Print and shaded views of the part. All mm, measured from the part's lowest x, y and z. Round coordinates to 2 decimals unless told otherwise and drop trailing zeros. Loops run counter-clockwise (first coordinate to the right, second up) from the corner with the lowest first, then second, coordinate; pieces in that order, holes last. Notation, with made-up numbers: (46, 6.5) - (93, 6.5) arc R25 cw to (93, 41.5) - close; hole circle Ø1 at (42, 2). An arc over 180 degrees is marked (long way). Use one line per item in the form item = value. Start each with the question number.
Q1. Saw through at B-B (y = 9.5). Give the cut face in (x, z), then the cut area to 3 significant figures.
Q2. Saw through at A-A (z = 37). Give the cut face in (x, y).
Q3. Saw through at C-C (x = 10). Give the cut face in (y, z), then the cut area to 3 significant figures.
Q4. Drill centre lines: line 1 (Z direction, x = 10, y = 5); line 2 (Z direction, x = 8.5, y = 9.25); line 3 (Z direction, x = 18.25, y = 8.75). Where is each one in solid material? Low to high.
Q5. Pin check, flat tips, straight feed: pin 1 (5 mm diameter, centred on y = 3, z = 33.5, fed in from -X); pin 2 (3.5 mm diameter, centred on x = 10, z = 37, fed in from +Y). Stop position of each tip, or through.
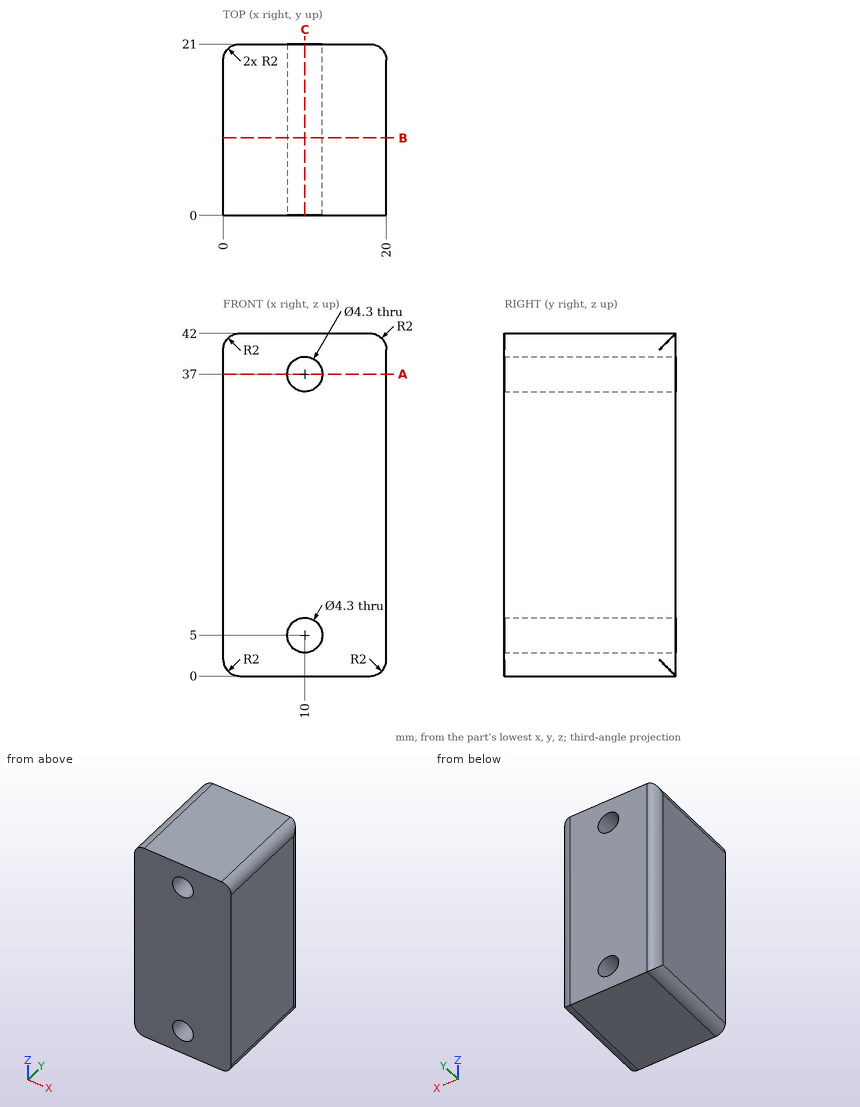
Report:
q1.outline = (0, 2) arc R2 ccw to (2, 0) - (18, 0) arc R2 ccw to (20, 2) - (20, 40) arc R2 ccw to (18, 42) - (2, 42) arc R2 ccw to (0, 40) - close; hole circle Ø4.3 at (10, 5); hole circle Ø4.3 at (10, 37)
q1.area = 808 mm²
q2.outline = (0, 0) - (7.85, 0) - (7.85, 21) - (2, 21) arc R2 ccw to (0, 19) - close; (12.15, 0) - (20, 0) - (20, 19) arc R2 ccw to (18, 21) - (12.15, 21) - close
q3.outline = (0, 0) - (21, 0) - (21, 2.85) - (0, 2.85) - close; (0, 7.15) - (21, 7.15) - (21, 34.85) - (0, 34.85) - close; (0, 39.15) - (21, 39.15) - (21, 42) - (0, 42) - close
q3.area = 701 mm²
q4.line_1 = 0 to 2.85, 7.15 to 34.85, 39.15 to 42
q4.line_2 = 0 to 3.46, 6.54 to 35.46, 38.54 to 42
q4.line_3 = 0.02 to 41.98
q5.pin_1 = 0
q5.pin_2 = through
